Can you work these out from the model? Positions are in its coordinate system, mm. Give positions to 0.01 mm unless a question says otherwise; leave off trailing zeros. Order: outer loops, then holes, each group sorted by start corner. A loop starts at its lowest first (then second) coordinate and runs counter-clockwise, first axis right, second up. Notation, with made-up numbers: M -18.75,40 L 39.25,40 A19 cw 39.25,56 Z; hole C -10.5,50 d7. An arc over 180 degrees is marked long. Answer as a JSON object with one key per item and string values.
```python
from build123d import *

# Parameters (mm, degrees)
CROQUIS1_W              = 9
CROQUIS1_H              = 6.5
SALIENTE_EXTRUIR1_DEPTH = 431
CROQUIS2_W              = 1.5
CROQUIS2_H              = 0.75
CORTAR_EXTRUIR1_DEPTH   = 431
CHAFL_N2_SIZE           = 0.5
CROQUIS3_R              = 1.8
CORTAR_EXTRUIR2_DEPTH   = 440
CHAFL_N4_SIZE           = 0.5
CROQUIS4_R              = 2.85
CORTAR_EXTRUIR3_DEPTH   = 4.4


with BuildPart() as part:
    # Croquis1 → Saliente-Extruir1 (new body)
    with BuildSketch(Plane(origin=(0, 0, 0), x_dir=(1, 0, 0), z_dir=(0, 1, 0))):
        with Locations((4.5, 3.25)):
            Rectangle(CROQUIS1_W, CROQUIS1_H)
    extrude(amount=SALIENTE_EXTRUIR1_DEPTH)

    # Croquis2 → Cortar-Extruir1 (cut)
    with BuildSketch(Plane(origin=(0, 431, 0), x_dir=(1, 0, 0), z_dir=(0, 1, 0))):
        with Locations((0.75, 4.375)):
            Rectangle(CROQUIS2_W, CROQUIS2_H)
        with Locations((8.25, 4.375)):
            Rectangle(CROQUIS2_W, CROQUIS2_H)
    extrude(amount=-CORTAR_EXTRUIR1_DEPTH, mode=Mode.SUBTRACT)

    # Chaflán2
    chafl_n2_edges = [part.edges().sort_by_distance(p)[0] for p in [
        (0, 215.5, -4.75),
        (0, 215.5, -4),
        (9, 215.5, -4.75),
        (9, 215.5, -4),
    ]]
    chamfer(chafl_n2_edges, length=CHAFL_N2_SIZE)

    # Croquis3 → Cortar-Extruir2 (cut)
    with BuildSketch(Plane.XY):
        with Locations((4.5, 415)):
            Circle(CROQUIS3_R)
        with Locations((4.5, 395)):
            Circle(CROQUIS3_R)
        with Locations((4.5, 375.052631579)):
            Circle(CROQUIS3_R)
        with Locations((4.5, 355.105263158)):
            Circle(CROQUIS3_R)
        with Locations((4.5, 335.157894737)):
            Circle(CROQUIS3_R)
        with Locations((4.5, 315.210526316)):
            Circle(CROQUIS3_R)
        with Locations((4.5, 295.263157895)):
            Circle(CROQUIS3_R)
        with Locations((4.5, 275.315789474)):
            Circle(CROQUIS3_R)
        with Locations((4.5, 255.368421053)):
            Circle(CROQUIS3_R)
        with Locations((4.5, 235.421052632)):
            Circle(CROQUIS3_R)
        with Locations((4.5, 215.473684211)):
            Circle(CROQUIS3_R)
        with Locations((4.5, 195.526315789)):
            Circle(CROQUIS3_R)
        with Locations((4.5, 175.578947368)):
            Circle(CROQUIS3_R)
        with Locations((4.5, 155.631578947)):
            Circle(CROQUIS3_R)
        with Locations((4.5, 135.684210526)):
            Circle(CROQUIS3_R)
        with Locations((4.5, 115.736842105)):
            Circle(CROQUIS3_R)
        with Locations((4.5, 95.789473684)):
            Circle(CROQUIS3_R)
        with Locations((4.5, 75.842105263)):
            Circle(CROQUIS3_R)
        with Locations((4.5, 55.894736842)):
            Circle(CROQUIS3_R)
        with Locations((4.5, 35.947368421)):
            Circle(CROQUIS3_R)
        with Locations((4.5, 16)):
            Circle(CROQUIS3_R)
    extrude(amount=-CORTAR_EXTRUIR2_DEPTH, mode=Mode.SUBTRACT)

    # Chaflán4
    chafl_n4_edges = [part.edges().sort_by_distance(p)[0] for p in [
        (4.5, 431, -6.5),
        (4.5, 0, -6.5),
        (4.5, 0, 0),
        (4.5, 431, 0),
        (0, 215.5, -6.5),
        (9, 215.5, -6.5),
        (9, 215.5, 0),
        (0, 215.5, 0),
    ]]
    chamfer(chafl_n4_edges, length=CHAFL_N4_SIZE)

    # Croquis4 → Cortar-Extruir3 (cut)
    with BuildSketch(Plane(origin=(0, 0, -6.5), x_dir=(-1, 0, 0), z_dir=(0, 0, -1))):
        with Locations((-4.5, 415)):
            Circle(CROQUIS4_R)
        with Locations((-4.5, 395.05)):
            Circle(CROQUIS4_R)
        with Locations((-4.5, 375.1)):
            Circle(CROQUIS4_R)
        with Locations((-4.5, 355.15)):
            Circle(CROQUIS4_R)
        with Locations((-4.5, 335.2)):
            Circle(CROQUIS4_R)
        with Locations((-4.5, 315.25)):
            Circle(CROQUIS4_R)
        with Locations((-4.5, 295.3)):
            Circle(CROQUIS4_R)
        with Locations((-4.5, 275.35)):
            Circle(CROQUIS4_R)
        with Locations((-4.5, 255.4)):
            Circle(CROQUIS4_R)
        with Locations((-4.5, 235.45)):
            Circle(CROQUIS4_R)
        with Locations((-4.5, 215.5)):
            Circle(CROQUIS4_R)
        with Locations((-4.5, 195.55)):
            Circle(CROQUIS4_R)
        with Locations((-4.5, 175.6)):
            Circle(CROQUIS4_R)
        with Locations((-4.5, 155.65)):
            Circle(CROQUIS4_R)
        with Locations((-4.5, 135.7)):
            Circle(CROQUIS4_R)
        with Locations((-4.5, 115.75)):
            Circle(CROQUIS4_R)
        with Locations((-4.5, 95.8)):
            Circle(CROQUIS4_R)
        with Locations((-4.5, 75.85)):
            Circle(CROQUIS4_R)
        with Locations((-4.5, 55.9)):
            Circle(CROQUIS4_R)
        with Locations((-4.5, 35.95)):
            Circle(CROQUIS4_R)
        with Locations((-4.5, 16)):
            Circle(CROQUIS4_R)
    extrude(amount=-CORTAR_EXTRUIR3_DEPTH, mode=Mode.SUBTRACT)


solid = part.part
```
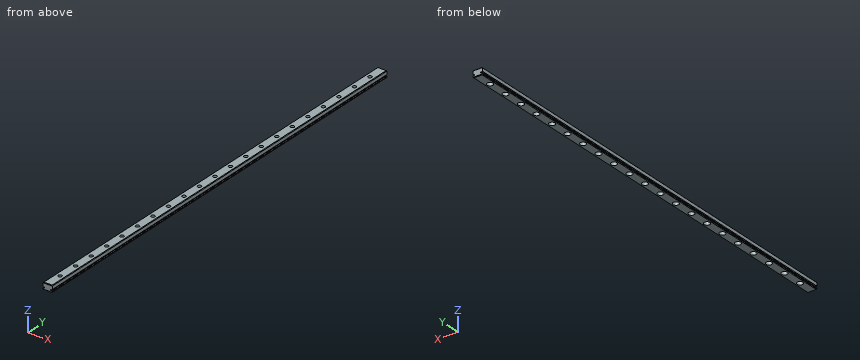
1) I want a section at A-A on y = 382.5. Write out the boundary of the cut face in (x, z).
Results found:
{"outline": "M 0,-6 L 0.5,-6.5 L 8.5,-6.5 L 9,-6 L 9,-5.25 L 8.5,-4.75 L 7.5,-4.75 L 7.5,-4 L 8.5,-4 L 9,-3.5 L 9,-0.5 L 8.5,0 L 0.5,0 L 0,-0.5 L 0,-3.5 L 0.5,-4 L 1.5,-4 L 1.5,-4.75 L 0.5,-4.75 L 0,-5.25 Z"}
2) I'm going to push flat-ended pins straight in: pin 1 Ø4.5 at (x, y) = (4.5, 135.7) entering from -Z; pin 2 Ø3 at (x, y) = (4.5, 135.68) entering from +Z; pin 3 Ø0.6 at (y, z) = (276.5, -4) entering from +X. Where does each tip first touch, or does it pass through?
Results found:
{"pin 1": "stops at z = -2.1", "pin 2": "passes through", "pin 3": "stops at x = 8.8"}
3) I need wall thicknesses on L1, parallel to X at y = 35.5, z = -3; L2, parallel to Z at x = 8, y = 76; L3, parallel to X at y = 172, z = -4.5. Which ranges of each line are inside material? Lowest first, please.
Results found:
{"L1": "x = 0 to 1.69, 7.31 to 9", "L2": "z = -6.5 to -4.75, -4 to 0", "L3": "x = 1.5 to 7.5"}
4) I want a section at B-B on x = 4.5. Count the separate pieces of the cut face and the enclosed holes in it, and give its area (3 significant figures).
Results found:
{"separate pieces": "22", "enclosed holes": "0", "area": "2,120 mm²"}
